Read the model definition and answer for the solid it produces. Units are mm, in the model's axes. A direction names the side the tool comes from. Coordinates: 2 decimals unless noted, no trailing zeros. Order: outer loops, then holes, each group sorted by start corner. A loop starts at its lowest first (then second) coordinate and runs counter-clockwise, first axis right, second up. Notation, with made-up numbers: M 3,42.25 L 53,42.25 A11 cw 53,62.25 Z; hole C 85,-6.75 d6. An arc over 180 degrees is marked long. Use a Markdown table: item, result. Add a question column.
1) Find section B-B on y = -13.5. Write down the section's boundary in (x, z), plus the area to 3 significant figures.
2) Find section A-A on x = -2.5. Write down the section's boundary in (y, z).
3) Find section D-D on y = -2.5. Write down the section's boundary in (x, z), plus the area to 3 significant figures.
4) For faces 1 (the face through (-44.5, 3, -1)), 2 (the face through (0, -15.3, -1)), 3 (the face through (41, -22, -1)), 4 (the face through (33, 23.5, -1)), determine the directions among +Z, -Z, +X, -X, +Y, -Y from which every point of the face is accessible in a straight line to the end or side of a thin tool.
5) Find section C-C on z = -0.7. Count the separate pieces of the cut face and the enclosed holes in it, plus the area to 3 significant figures.
6) The mould has two halves that part along Y. Classify faces 5 (the face through (6, -3, -1)), 6 (the face through (1, 2, 0)), 7 (the face through (26, -23.5, -1)): released by +Y, released by -Y, zero draft, split by the parting line, or undercut.
7) Each of these flat-tipped pins is pushed along its axis until it touches: pin 1 Ø0.8 at (x, z) = (-45.5, -1) entering from +Y; pin 2 Ø0.6 at (y, z) = (4, -1) entering from +X; pin 3 Ø0.6 at (y, z) = (-3, -1) entering from -X. Where does it stop, or does it pass through?
8) Find the intervals of material crossed by probe 1 along Y at (x, z) = (-3, -0.8); probe 2 along X at (y, z) = (-1.5, -1); probe 3 along Y at (x, z) = (9, -1.1), in increasing order. Write a range as [from, to].
from build123d import *

# Parameters (mm, degrees)
BOSS_EXTRUDE1_DEPTH = 2.1
SKETCH2_W           = 28
SKETCH2_H           = 4.5
SKETCH2_W_2         = 12
SKETCH2_H_2         = 8
CUT_EXTRUDE2_DEPTH  = 54.128711635
SKETCH3_W           = 1.5
SKETCH3_H           = 17
SKETCH3_W_2         = 10
SKETCH3_H_2         = 1.5
SKETCH3_W_3         = 32
CUT_EXTRUDE3_DEPTH  = 54.128711635


with BuildPart() as part:
    # Sketch1 → Boss-Extrude1 (new body)
    with BuildSketch(Plane.XY):
        Polygon((-46, 23.5), (-20.5, 23.5), (-20.5, 26.5), (20.5, 26.5), (20.5, 23.5), (46, 23.5), (46, -23.5), (-46, -23.5), align=None)
    extrude(amount=-BOSS_EXTRUDE1_DEPTH)

    # Sketch2 → Cut-Extrude2 (cut, through all)
    with BuildSketch(Plane.XY):
        with Locations((0, -13.05)):
            Rectangle(SKETCH2_W, SKETCH2_H)
        with Locations((0, -2.8)):
            Rectangle(SKETCH2_W_2, SKETCH2_H_2)
    extrude(amount=-CUT_EXTRUDE2_DEPTH, mode=Mode.SUBTRACT)

    # Sketch3 → Cut-Extrude3 (cut, through all)
    with BuildSketch(Plane.XY):
        with Locations((-45.25, 3)):
            Rectangle(SKETCH3_W, SKETCH3_H)
        with Locations((-41, -22.75)):
            Rectangle(SKETCH3_W_2, SKETCH3_H_2)
        with Locations((0, -22.75)):
            Rectangle(SKETCH3_W_3, SKETCH3_H_2)
        with Locations((41, -22.75)):
            Rectangle(SKETCH3_W_2, SKETCH3_H_2)
        with Locations((45.25, 3)):
            Rectangle(SKETCH3_W, SKETCH3_H)
    extrude(amount=-CUT_EXTRUDE3_DEPTH, mode=Mode.SUBTRACT)


solid = part.part
Check result:
| question | item | result |
|---|---|---|
| 1 | outline | M -46,-2.1 L -14,-2.1 L -14,0 L -46,0 Z; M 14,-2.1 L 46,-2.1 L 46,0 L 14,0 Z |
| 1 | area | 134 mm2 |
| 2 | outline | M -22,-2.1 L -15.3,-2.1 L -15.3,0 L -22,0 Z; M -10.8,-2.1 L -6.8,-2.1 L -6.8,0 L -10.8,0 Z; M 1.2,-2.1 L 26.5,-2.1 L 26.5,0 L 1.2,0 Z |
| 3 | outline | M -44.5,-2.1 L -6,-2.1 L -6,0 L -44.5,0 Z; M 6,-2.1 L 44.5,-2.1 L 44.5,0 L 6,0 Z |
| 3 | area | 162 mm2 |
| 4 | face 1 | +Z, -Z, -X |
| 4 | face 2 | +Z, -Z |
| 4 | face 3 | +Z, -Z, +X, -Y |
| 4 | face 4 | +Z, -Z, +X, +Y |
| 5 | separate pieces | 1 |
| 5 | enclosed holes | 2 |
| 5 | area | 4,100 mm2 |
| 6 | face 5 | undercut |
| 6 | face 6 | zero draft |
| 6 | face 7 | released by -Y |
| 7 | pin 1 | stops at y = 23.5 |
| 7 | pin 2 | stops at x = 44.5 |
| 7 | pin 3 | stops at x = -44.5 |
| 8 | probe 1 | y = [-22, -15.3], [-10.8, -6.8], [1.2, 26.5] |
| 8 | probe 2 | x = [-44.5, -6], [6, 44.5] |
| 8 | probe 3 | y = [-22, -15.3], [-10.8, 26.5] |
